from build123d import *

# Parameters (mm, degrees)
F0_W     = 12.7625
F0_H     = 76.2625
F0_R     = 4
F0_R_2   = 1.35255
F0_W_2   = 8
F0_H_2   = 42.8
F1_DEPTH = 6.35
F2_R     = 0.79375
F3_SIZE  = 0.254
F4_R     = 1.35255
F5_DEPTH = 2.38125


with BuildPart() as f1:
    # F0 (on Top) → F1 (new body)
    with BuildSketch(Plane.XY):
        Rectangle(F0_W, F0_H)
        with Locations((0, -31.75)):
            Circle(F0_R, mode=Mode.SUBTRACT)
        with Locations((0, -24.575)):
            Circle(F0_R_2, mode=Mode.SUBTRACT)
        Rectangle(F0_W_2, F0_H_2, mode=Mode.SUBTRACT)
        with Locations((0, 24.575)):
            Circle(F0_R_2, mode=Mode.SUBTRACT)
        with Locations((0, 31.75)):
            Circle(F0_R, mode=Mode.SUBTRACT)
    extrude(amount=F1_DEPTH)

    # F2
    f2_edges = [f1.edges().sort_by_distance(p)[0] for p in [
        (4, -21.4, 3.175),
        (-4, -21.4, 3.175),
        (-4, 21.4, 3.175),
        (4, 21.4, 3.175),
    ]]
    fillet(f2_edges, radius=F2_R)

    # F3
    f3_edges = [f1.edges().sort_by_distance(p)[0] for p in [
        (-4, 31.75, 6.35),
        (-4, -31.75, 6.35),
    ]]
    chamfer(f3_edges, length=F3_SIZE)

    # F4 (on face) → F5 (cut, through all)
    with BuildSketch(Plane.YZ.offset(6.38125)):
        with Locations((-18.225, 3.175)):
            Circle(F4_R)
        with Locations((18.225, 3.175)):
            Circle(F4_R)
    extrude(amount=-F5_DEPTH, mode=Mode.SUBTRACT)


solid = f1.part
Input: part model. Units: mm. Frame: model coordinates. A direction names the side the tool comes from. Give positions to 0.01 mm unless a question says otherwise; leave off trailing zeros. Order: outer loops, then holes, each group sorted by start corner. A loop starts at its lowest first (then second) coordinate and runs counter-clockwise, first axis right, second up. Notation, with made-up numbers: (57.5, 52) - (116.5, 52) arc R12 cw to (116.5, 61) - close; hole circle Ø11 at (-22.5, 1). An arc over 180 degrees is marked (long way). Answer as a JSON object with one key per item and string values. Group by question number.
Q1. Cut plane A-A, the plane y = -12. Output: boundary loops of the cut face in (x, z), then the cut area to 3 significant figures.
Q2. First-contact query: pin 1 Ø5 at (x, y) = (0, -31.75) entering from +Z. Flat tip, straight axial feed; report the tip coordinate or a pass-through.
Q3. Cut plane C-C, the plane x = 0. Output: boundary loops of the cut face in (y, z).
Q4. Cut plane D-D, the plane y = -31.75. Output: boundary loops of the cut face in (x, z).
Q5. Set-up query: faces 1 (the face through (5.207, 16.874, 3.234)), 2 (the face through (-4, 0, 3)), 3 (the face through (6.381, -1, 3)). Return all of +Z, -Z, +X, -X, +Y, -Y with unobstructed straight access to the full face (end or side cutting, diameter ignored); none if empty.
Q6. Cut plane B-B, the plane z = 2.5. Count the separate pieces of the cut face and the enclosed holes in it, then the cut area to 3 significant figures.
Q7. Mould query, pull axis Y, two halves, no side actions, for faces 4 (the face through (-4.3, 0.5, 0)), 5 (the face through (0, 38.131, 3)), 6 (the face through (5.207, -19.576, 3.234)). Classes: pulls with the +Y half, pulls with the -Y half, needs draft (parallel to the pull), parting line crosses it, or undercut.
Q8. Line query: probe 1 along Y at (x, z) = (0, 2.5); probe 2 along X at (y, z) = (-12.5, 2.5); probe 3 along Y at (x, z) = (2.25, 5.5). Output: solid intervals per line, ascending.
Results:
{
 "1": {"outline": "(-6.38, 0) - (-4, 0) - (-4, 6.35) - (-6.38, 6.35) - close; (4, 0) - (6.38, 0) - (6.38, 6.35) - (4, 6.35) - close", "area": "30.2 mm^2"},
 "2": {"pin 1": "through"},
 "3": {"outline": "(-38.13, 0) - (-35.75, 0) - (-35.75, 6.1) - (-36, 6.35) - (-38.13, 6.35) - close; (-27.75, 0) - (-25.93, 0) - (-25.93, 6.35) - (-27.5, 6.35) - (-27.75, 6.1) - close; (-23.22, 0) - (-21.4, 0) - (-21.4, 6.35) - (-23.22, 6.35) - close; (21.4, 0) - (23.22, 0) - (23.22, 6.35) - (21.4, 6.35) - close; (25.93, 0) - (27.75, 0) - (27.75, 6.1) - (27.5, 6.35) - (25.93, 6.35) - close; (35.75, 0) - (38.13, 0) - (38.13, 6.35) - (36, 6.35) - (35.75, 6.1) - close"},
 "4": {"outline": "(-6.38, 0) - (-4, 0) - (-4, 6.1) - (-4.25, 6.35) - (-6.38, 6.35) - close; (4, 0) - (6.38, 0) - (6.38, 6.35) - (4.25, 6.35) - (4, 6.1) - close"},
 "5": {"face 1": "+X", "face 2": "+Z, -Z", "face 3": "+Z, -Z, +X, +Y, -Y"},
 "6": {"separate pieces": "2", "enclosed holes": "4", "area": "508 mm^2"},
 "7": {"face 4": "needs draft", "face 5": "pulls with the +Y half", "face 6": "undercut"},
 "8": {"probe 1": "-38.13 to -35.75, -27.75 to -25.93, -23.22 to -21.4, 21.4 to 23.22, 25.93 to 27.75, 35.75 to 38.13", "probe 2": "-6.38 to -4, 4 to 6.38", "probe 3": "-38.13 to -35.06, -28.44 to -21.4, 21.4 to 28.44, 35.06 to 38.13"}
}
